Can you work these out from the model? Positions are in its coordinate system, mm. Face numbers are marked on the shaded views. A direction names the side the tool comes from. Round coordinates to 2 decimals unless told otherwise and drop trailing zeros. Loops run counter-clockwise (first coordinate to the right, second up) from the corner with the lowest first, then second, coordinate; pieces in that order, holes last. Notation, with made-up numbers: (49.25, 27) -> (89.25, 27) arc R26 cw to (89.25, 48) -> close; hole circle Ø10 at (9, -32.75). An arc over 180 degrees is marked (long way). Use a Markdown table: item, result.
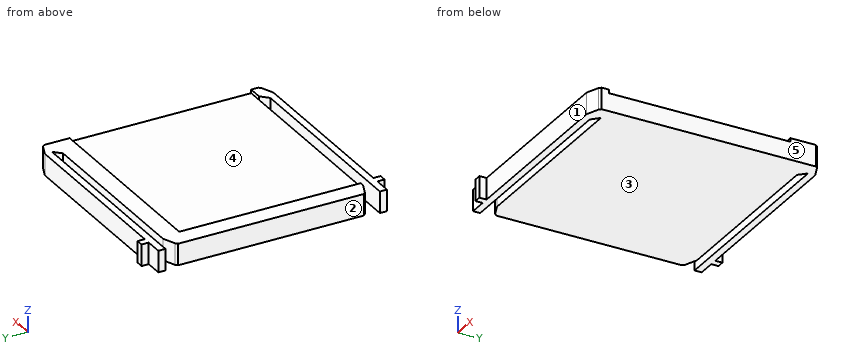
Autodesk Inventor part; units mm, degrees
ref_plane "Work Plane1" through (2, 15, 3) normal (0, -1, 0) x (1, 0, 0)
ref_plane "YZ Plane" through (0, 0, 0) normal (1, 0, 0) x (0, 1, 0)
ref_plane "XZ Plane" through (0, 0, 0) normal (0, 1, 0) x (-1, 0, 0)
sketch "Sketch1" plane through (0, 0, 0) normal (0, 0, 1) x (1, 0, 0)
  line L0 (0, 0) -> (30, 0)
  line L1 (30, 0) -> (30, 30)
  line L2 (30, 30) -> (0, 30)
  line L3 (0, 30) -> (0, 0)
  dimension "d0" = 30
  dimension "d1" = 30
extrude "Extrusion1" add sketch "Sketch1" along normal blind 3
sketch "Sketch2" plane through (0, 0, 3) normal (0, 0, 1) x (1, 0, 0)
  line L0 (30, 3.6) -> (2.6, 3.6)
  line L1 (2.6, 3.6) -> (2.6, 29)
  line L2 (2.6, 29) -> (30, 29)
  line L3 (30, 29) -> (30, 3.6)
  line L4 (0, 0) -> (30, 0)
  line L5 (30, 0) -> (30, 30)
  dimension "d4" = 27.4
  dimension "d5" = 25.4
  dimension "d36" = 3.6
extrude "Extrusion2" cut sketch "Sketch2" against normal blind 0.5
sketch "Sketch3" plane through (0, 0, 3) normal (0, 0, 1) x (1, 0, 0)
  line L0 (30, 30) -> (0, 30)
  line L1 (0, 30) -> (0, 0)
  line L2 (28, 30) -> (0, 30)
  line L3 (0, 30) -> (0, 29)
  line L4 (0, 29) -> (28, 29)
  line L5 (28, 29) -> (28, 30)
  line L6 (30, 29) -> (30, 30)
  line L7 (0, 0) -> (30, 0)
  line L8 (28, 0) -> (0, 0)
  line L9 (0, 0) -> (0, 1)
  line L10 (0, 1) -> (28, 1)
  line L11 (28, 1) -> (28, 0)
  line L12 (30, 0) -> (30, 3.6)
  dimension "d8" = 1
  dimension "d9" = 2
  dimension "d10" = 1
  dimension "d11" = 2
extrude "Extrusion3" cut sketch "Sketch3" against normal through all
sketch "Sketch4" plane through (0, 0, 3) normal (0, 0, 1) x (1, 0, 0)
  line L0 (30, 29) -> (30, 30)
  line L1 (30, 30) -> (-0.4, 30)
  line L2 (-0.4, 30) -> (-0.4, 31)
  line L3 (-0.4, 31) -> (30, 31)
  line L4 (30, 31) -> (30, 30)
  line L5 (30, 0) -> (-0.4, 0)
  line L6 (-0.4, 0) -> (-0.4, -1)
  line L7 (-0.4, -1) -> (30, -1)
  line L8 (30, -1) -> (30, 0)
  line L9 (2, 31) -> (3, 31)
  line L10 (3, 31) -> (3, 32)
  line L11 (3, 32) -> (2, 32)
  line L12 (2, 32) -> (2, 31)
  line L13 (2, -1) -> (3, -1)
  line L14 (3, -1) -> (3, -2)
  line L15 (3, -2) -> (2, -2)
  line L16 (2, -2) -> (2, -1)
  line L17 (0, 29) -> (0, 1)
  point P0 (0, 0)
  dimension "d14" = 30.4
  dimension "d15" = 1
  dimension "d17" = 1
  dimension "d20" = 1
  dimension "d21" = 1
  dimension "d26" = 1
  dimension "d27" = 1
  dimension "d35" = 2
extrude "Extrusion4" add sketch "Sketch4" against normal blind 3
chamfer "Chamfer1" distance 1 angle 45 4 edges at (30, 31, 1.5) (30, -1, 1.5) (28, 1, 1.5) (28, 30, 1.5)
chamfer "Chamfer2" distance 1 angle 45 2 edges at (29.0001, 31, 1.5) (29.0001, -1, 1.5)
ref_plane "Work Plane1" through (2, 15, 3) normal (0, -1, 0) x (1, 0, 0)
mirror "Mirror1" about plane through (2, 15, 3) normal (0, -1, 0) of "Extrusion1", "Extrusion2", "Extrusion3", "Extrusion4", "Chamfer1", "Chamfer2"
chamfer "Chamfer3" distance 1 angle 45 2 edges at (0, 29, 1.5) (0, 1, 1.5)
chamfer "Chamfer4" distance 1 angle 45 2 edges at (1, 29, 1.5) (1, 1, 1.5)
properties part number "TA10" material "ABS Plastic"
1. I want a section at A-A (x = 24.5). Please give me the cut outline in (y, z).
Answer sheet:
| item | result |
|---|---|
| outline | (-1, 0) -> (0, 0) -> (0, 3) -> (-1, 3) -> close; (1, 0) -> (29, 0) -> (29, 3) -> (26.4, 3) -> (26.4, 2.5) -> (1, 2.5) -> close; (30, 0) -> (31, 0) -> (31, 3) -> (30, 3) -> close |
2. Will these pins go through, and if not, where does the flat tip stop? pin 1 Ø1.5 at (x, z) = (15, 1.5) entering from -Y; pin 2 Ø0.6 at (y, z) = (8, 3) entering from +X; pin 3 Ø1.1 at (y, z) = (31.5, 1) entering from +X; pin 4 Ø1 at (x, y) = (26.5, 21.5) entering from -Z.
Answer sheet:
| item | result |
|---|---|
| pin 1 | stops at y = -1 |
| pin 2 | stops at x = 2.6 |
| pin 3 | stops at x = 28.12 |
| pin 4 | stops at z = 0 |
3. I want a section at B-B (y = 17.5). Please give me the cut outline in (x, z).
Answer sheet:
| item | result |
|---|---|
| outline | (0, 0) -> (30, 0) -> (30, 2.5) -> (2.6, 2.5) -> (2.6, 3) -> (0, 3) -> close |
4. Which directions (+Z, -Z, +X, -X, +Y, -Y) give clear straight access to the entire face, cutting with the end or side of a thin tool? Please do the marked faces 4 and 5.
Answer sheet:
| item | result |
|---|---|
| face 4 | +Z, +X |
| face 5 | +Z, -Z, +X, +Y, -Y |
5. If we mould it in two halves opening along Y, with no side actions, what happens to the marked faces 1, 2 and 3? For each: +Y half, -Y half, draft (parallel to the pull), parting line (faces both ways), or undercut.
Answer sheet:
| item | result |
|---|---|
| face 1 | -Y half |
| face 2 | undercut |
| face 3 | draft |
6. I need wall thicknesses on line 1 (Y direction, x = 19.5, z = 1.25); line 2 (Y direction, x = 23, z = 2.7); line 3 (Z direction, x = 11, y = 20). Which ranges of each line are inside material? Lowest first, please.
Answer sheet:
| item | result |
|---|---|
| line 1 | y = -1 to 0, 1 to 29, 30 to 31 |
| line 2 | y = -1 to 0, 26.4 to 29, 30 to 31 |
| line 3 | z = 0 to 2.5 |
